Autodesk Inventor part; units mm, degrees
ref_plane "YZ Plane" through (0, 0, 0) normal (1, 0, 0) x (0, 1, 0)
ref_plane "XZ Plane" through (0, 0, 0) normal (0, 1, 0) x (-1, 0, 0)
ref_plane "XY Plane" through (0, 0, 0) normal (0, 0, 1) x (1, 0, 0)
sketch "スケッチ1" plane through (0, 0, 0) normal (1, 0, 0) x (0, 1, 0)
  circle A0 centre (0, 0) radius 28
  line L0 (16.8575, 19.7946) -> (16.8575, -19.7946)
  line L1 (14.8575, 18.8482) -> (14.8575, -18.8482)
  arc A1 (18.1557, 18.611) -> (18.8392, -17.9188) centre (0, 0) ccw
  arc A2 (14.8575, 18.8482) -> (14.8575, -18.8482) centre (0, 0) ccw
  arc A3 (16.8575, 19.7946) -> (18.1557, 18.611) centre (0, 0) ccw
  arc A4 (18.8392, -17.9188) -> (16.8575, -19.7946) centre (0, 0) ccw
  line L2 (16.8575, 19.7946) -> (16.8575, -19.7946)
  line L3 (21.8575, 17.5) -> (21.8575, -17.5)
  dimension "d0" = 56
  dimension "d1" = 2
  dimension "d2" = 2
  dimension "d3" = 2
  dimension "d4" = 35
  dimension "d5" = 5
extrude "押し出し1" add sketch "スケッチ1" against normal blind 2 contours A0 L3 A3 | L3 A3 A1 A0 | L3 A3 A1 L0 | A3 L3 | L0 A1 | L1 A2
extrude "押し出し2" add sketch "スケッチ1" along normal blind 2 contours L0 A1
sketch "スケッチ2" plane through (0, 0, 0) normal (1, 0, 0) x (0, 0, -1)
  circle A0 centre (0, 0) radius 3.75
  circle A1 centre (0, 0) radius 7.5
  dimension "d10" = 7.5
  dimension "d11" = 15
extrude "押し出し3" cut sketch "スケッチ2" against normal blind 2 contours A0
extrude "押し出し4" add sketch "スケッチ2" along normal blind 2
sketch "スケッチ3" plane through (2, 0, 0) normal (1, 0, 0) x (0, 0, -1)
  circle A0 centre (0, 0) radius 6
  dimension "d16" = 12
extrude "押し出し5" cut sketch "スケッチ3" against normal blind 2.9
sketch "スケッチ4" plane through (0, 0, 0) normal (1, 0, 0) x (0, 0, -1)
  circle A0 centre (-10.8, 0) radius 3
  circle A1 centre (10.8, 0) radius 3
  circle A2 centre (-10.8, 0) radius 1.5
  circle A3 centre (10.8, 0) radius 1.5
  circle A4 centre (0, 0) radius 3.75
  dimension "d19" = 6
  dimension "d20" = 6
  dimension "d21" = 3
  dimension "d22" = 3
  dimension "d23" = 10.8
  dimension "d25" = 21.6
  dimension "d26" = 10.8
extrude "押し出し6" add sketch "スケッチ4" along normal blind 9.5 contours A0 | A1
properties part number "turn2Part"
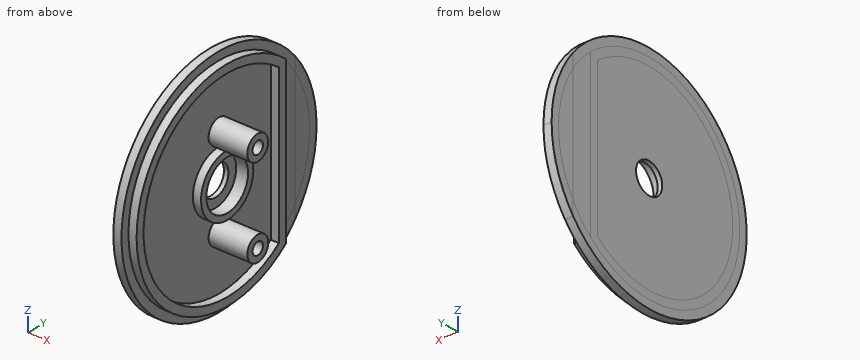
Geometry check sheet. Reference: the model listing, model coordinates, mm. Give positions to 0.01 mm unless a question says otherwise; leave off trailing zeros. Loops run counter-clockwise (first coordinate to the right, second up) from the corner with the lowest first, then second, coordinate; pieces in that order, holes last. Notation, with made-up numbers: M 41,21 L 58,21 A6 ccw 58,32 Z; hole C -36.75,20.25 d10. An arc over 180 degrees is marked long. Write item = value, one per line. Start each with the question number.
1. Thickness scan on probe 1 along Y at (x, z) = (0.65, 0); probe 2 along Y at (x, z) = (0.5, 10.5); probe 3 along X at (y, z) = (-6, -7). Record the ranges inside material, lowest first.
2. Go/stop test with flat-tipped pins: P1, Ø2.5, axis at y = 0.5, z = 11.5, coming from the +X side; P2, Ø3, axis at x = 0, z = -20.5, coming from the +Y side; P3, Ø1, axis at y = -4.5, z = -13, coming from the +X side; P4, Ø4.5, axis at y = -1, z = 3, coming from the +X side. Record where each tip stops, or that it passes through.
3. Section check D-D, the plane z = -20.5. Enter the section's corners in (x, y).
4. Section check A-A, the plane x = 1. Enter the section's corners in (y, z), plus the area to 3 significant figures.
5. Section check C-C, the plane y = -13. Enter the section's corners in (x, z), plus the area to 3 significant figures.
6. Section check B-B, the plane x = 7.75. Enter the section's corners in (y, z).
Values follow:
q1.probe_1 = -26 to -24, -7.5 to -6, 6 to 7.5, 14.86 to 16.86
q1.probe_2 = -23.79 to -21.58, -2.98 to -1.47, 1.47 to 2.98, 14.86 to 16.86
q1.probe_3 = -2 to 0
q2.P1 = 9.5
q2.P2 = 20.57
q2.P3 = 0
q2.P4 = -0.9
q3.outline = M -2,-19.07 L 0,-19.07 L 0,-15.99 L 2,-15.99 L 2,-12.48 L 0,-12.48 L 0,12.48 L 2,12.48 L 2,15.99 L 0,15.99 L 0,19.07 L -2,19.07 Z
q4.outline = C 0,0 d15; C 0,-10.8 d6; C 0,10.8 d6; M 16.86,-19.79 L 16.86,19.79 A26 ccw long Z; hole C 0,0 d12; hole C 0,-10.8 d3; hole C 0,10.8 d3; hole M 14.86,-18.85 L 14.86,18.85 A24 ccw long Z
q4.area = 409 mm^2
q5.outline = M -2,-24.8 L 0,-24.8 L 0,-22.52 L 2,-22.52 L 2,-20.17 L 0,-20.17 L 0,20.17 L 2,20.17 L 2,22.52 L 0,22.52 L 0,24.8 L -2,24.8 Z
q5.area = 109 mm^2
q6.outline = C 0,-10.8 d6; C 0,10.8 d6; hole C 0,-10.8 d3; hole C 0,10.8 d3
